Input: part model. Units: mm. Frame: model coordinates. Coordinates: 2 decimals unless noted, no trailing zeros. Loops run counter-clockwise (first coordinate to the right, second up) from the corner with the lowest first, then second, coordinate; pieces in that order, holes last.
(1) Contact query for flat-ended pins moving along their axis: P1, Ø4, axis at y = 1.5, z = -14.5, coming from the -X side; P2, Ø4, axis at y = 7.5, z = -11.5, coming from the +X side; P3, Ø6, axis at y = 6.5, z = 1, coming from the +X side. Output: stop coordinate, or through.
(2) Line query: L1, parallel to X at y = 6, z = 0; L2, parallel to X at y = 2.25, z = 5.5; L3, parallel to Z at x = -128.5, y = 6.25. Output: solid intervals per line, ascending.
(3) Section D-D, the plane z = -17. Return loops of the section in (x, y), then the cut area to 3 significant figures.
(4) Section B-B, the plane y = 8.5. Return loops of the section in (x, z).
(5) Section C-C, the plane z = 9. Return loops of the section in (x, y), then the cut area to 3 significant figures.
(6) Section A-A, the plane z = 0. Return loops of the section in (x, y).
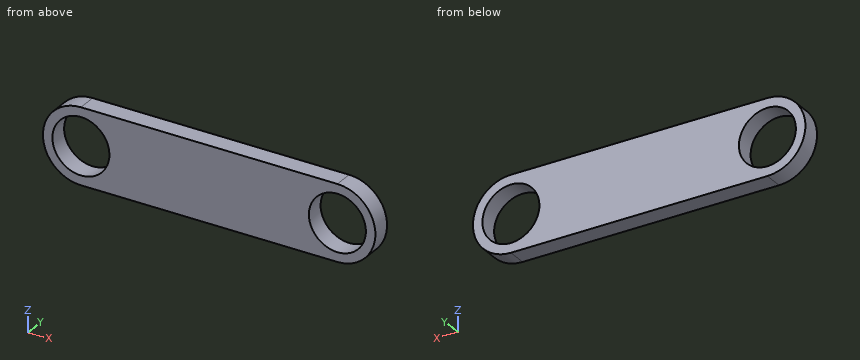
```python
from build123d import *

# Parameters (mm, degrees)
SKETCH1_R           = 15
BOSS_EXTRUDE1_DEPTH = 10
SKETCH2_R           = 15
CUT_EXTRUDE1_DEPTH  = 10


with BuildPart() as part:
    # Sketch1 → Boss-Extrude1 (new body)
    with BuildSketch(Plane(origin=(0, 0, 0), x_dir=(1, 0, 0), z_dir=(0, 1, 0))):
        with BuildLine():
            Line((-134.186746988, 20), (0.813253012, 20))
            ThreePointArc((0.813253012, 20), (20.813253012, 0), (0.813253012, -20))
            Line((0.813253012, -20), (-134.186746988, -20))
            ThreePointArc((-134.186746988, -20), (-154.186746988, 0), (-134.186746988, 20))
        make_face()
        with Locations(Location((-134.186746988, 0, 0), (0, 0, 270))):
            Circle(SKETCH1_R, mode=Mode.SUBTRACT)
    extrude(amount=BOSS_EXTRUDE1_DEPTH)

    # Sketch2 → Cut-Extrude1 (cut)
    with BuildSketch(Plane(origin=(0, 10, 0), x_dir=(1, 0, 0), z_dir=(0, 1, 0))):
        with Locations(Location((0.813253012, 0, 0), (0, 0, 270))):
            Circle(SKETCH2_R)
    extrude(amount=-CUT_EXTRUDE1_DEPTH, mode=Mode.SUBTRACT)


solid = part.part
```
Report:
1. P1: stops at x = -149.8
1. P2: stops at x = 18.41
1. P3: stops at x = 20.81
2. L1: x = -154.19 to -149.19, -119.19 to -14.19, 15.81 to 20.81
2. L2: x = -153.42 to -148.14, -120.23 to -13.14, 14.77 to 20.04
2. L3: z = -20 to -13.88, 13.88 to 20
3. outline: (-144.72, 0) - (11.35, 0) - (11.35, 10) - (-144.72, 10) - close
3. area: 1,560 mm2
4. outline: (-134.19, -20) - (0.81, -20) arc R20 ccw to (0.81, 20) - (-134.19, 20) arc R20 ccw to start; hole circle Ø30 at (-134.19, 0); hole circle Ø30 at (0.81, 0)
5. outline: (-152.05, 0) - (-146.19, 0) - (-146.19, 10) - (-152.05, 10) - close; (-122.19, 0) - (-11.19, 0) - (-11.19, 10) - (-122.19, 10) - close; (12.81, 0) - (18.67, 0) - (18.67, 10) - (12.81, 10) - close
5. area: 1,230 mm2
6. outline: (-154.19, 0) - (-149.19, 0) - (-149.19, 10) - (-154.19, 10) - close; (-119.19, 0) - (-14.19, 0) - (-14.19, 10) - (-119.19, 10) - close; (15.81, 0) - (20.81, 0) - (20.81, 10) - (15.81, 10) - close
